Here's how the part is built. I have some questions about the finished solid (model axes, mm). Face numbers are marked on the shaded views. Round coordinates to 2 decimals unless told otherwise and drop trailing zeros. Order: outer loops, then holes, each group sorted by start corner. A loop starts at its lowest first (then second) coordinate and runs counter-clockwise, first axis right, second up. Notation, with made-up numbers: (-40, -23.5) -> (-25, -23.5) arc R24 cw to (-25, 3.5) -> close; hole circle Ø3 at (-11, 4.25). An arc over 180 degrees is marked (long way). Use a Markdown table: item, result. Add a question column.
(1) If I drill on probe 1 along X at (y, z) = (3, 0.3); probe 2 along X at (y, z) = (1.5, 2.8); probe 3 along Y at (x, z) = (-4, 0.45), over which ranges is the centre line in solid material (lowest first)?
(2) I want a section at B-B, the plane z = 2.4. Please give me the cut outline in (x, y).
(3) Thinking about a two-plate mould opening in Y: for the marked faces 1, 2 and 3, which applies, pulls with the +Y half, pulls with the -Y half, needs draft (parallel to the pull), parting line crosses it, or undercut?
(4) I want a section at C-C, the plane y = 3.5. Please give me the cut outline in (x, z).
(5) I'm going to push a flat-ended pin straight in: P1, Ø2.5, axis at x = -5.36, y = 2.7, coming from the -Z side (1 decimal). Where does the tip first touch, or does it pass through?
(6) I want a section at A-A, the plane y = 2.25. Please give me the cut outline in (x, z), then the cut area to 3 significant figures.
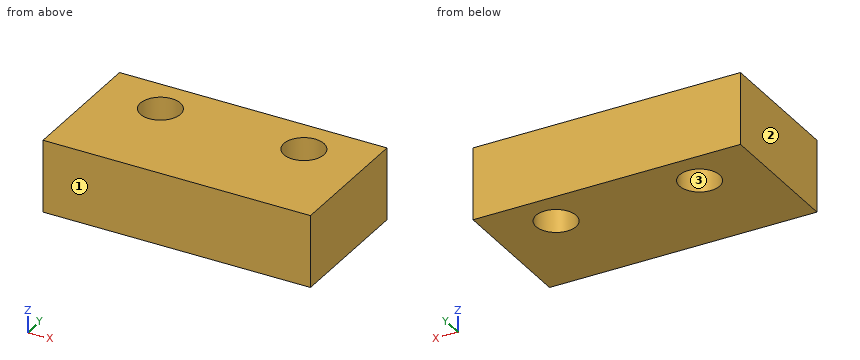
Autodesk Inventor part; units mm, degrees
ref_plane "YZ Plane" through (0, 0, 0) normal (1, 0, 0) x (0, 1, 0)
ref_plane "XZ Plane" through (0, 0, 0) normal (0, 1, 0) x (-1, 0, 0)
ref_plane "XY Plane" through (0, 0, 0) normal (0, 0, 1) x (1, 0, 0)
sketch "草图1" plane through (0, 0, 0) normal (0, 0, 1) x (1, 0, 0)
  line L0 (10, -4.6392) -> (-10, -4.6392)
  line L1 (-10, -4.6392) -> (-10, 5.5)
  line L2 (-10, 5.5) -> (10, 5.5)
  line L3 (10, 5.5) -> (10, -4.6392)
  point P0 (0, 0)
  dimension "d0" = 20
  dimension "d7" = 10.1392
extrude "拉伸1" add sketch "草图1" along normal blind 5.4
sketch "草图2" plane through (0, 0, 5.4) normal (0, 0, 1) x (1, 0, 0)
  circle A0 centre (-5.3642, 2.7045) radius 1.5
  circle A1 centre (5.3642, 2.7045) radius 1.5
  point P0 (0, 0)
extrude "拉伸2" cut sketch "草图2" against normal blind 21.65
properties part number "攻单夹片"
Taken from the geometry:
| question | item | result |
|---|---|---|
| 1 | probe 1 | x = -10 to -6.83, -3.89 to 3.89, 6.83 to 10 |
| 1 | probe 2 | x = -10 to -6.26, -4.47 to 4.47, 6.26 to 10 |
| 1 | probe 3 | y = -4.64 to 2.08, 3.33 to 5.5 |
| 2 | outline | (-10, -4.64) -> (10, -4.64) -> (10, 5.5) -> (-10, 5.5) -> close; hole circle Ø3 at (-5.36, 2.7); hole circle Ø3 at (5.36, 2.7) |
| 3 | face 1 | pulls with the -Y half |
| 3 | face 2 | needs draft |
| 3 | face 3 | undercut |
| 4 | outline | (-10, 0) -> (-6.64, 0) -> (-6.64, 5.4) -> (-10, 5.4) -> close; (-4.09, 0) -> (4.09, 0) -> (4.09, 5.4) -> (-4.09, 5.4) -> close; (6.64, 0) -> (10, 0) -> (10, 5.4) -> (6.64, 5.4) -> close |
| 5 | P1 | passes through |
| 6 | outline | (-10, 0) -> (-6.79, 0) -> (-6.79, 5.4) -> (-10, 5.4) -> close; (-3.93, 0) -> (3.93, 0) -> (3.93, 5.4) -> (-3.93, 5.4) -> close; (6.79, 0) -> (10, 0) -> (10, 5.4) -> (6.79, 5.4) -> close |
| 6 | area | 77.1 mm2 |
